from build123d import *

# Parameters (mm, degrees)
BOSS_EXTRUDE1_DEPTH = 13.33
FILLET1_R           = 20
SKETCH3_R           = 3.33
CUT_EXTRUDE2_DEPTH  = 68.320131462
FILLET2_R           = 3.333
SKETCH4_R           = 2.8333333
DOME1_FACE_RADIUS   = 2.8333333
DOME1_HEIGHT        = 3.3333333
CUT_EXTRUDE3_DEPTH  = 2
CUT_EXTRUDE5_DEPTH  = 13.34
SKETCH19_R          = 1.425
CUT_EXTRUDE6_DEPTH  = 8.6


with BuildPart() as part:
    # Sketch1 → Boss-Extrude1 (new body)
    with BuildSketch(Plane(origin=(0, 0, 0), x_dir=(1, 0, 0), z_dir=(0, 1, 0))):
        with BuildLine():
            Line((25.438564969, 21.535280641), (27.993333135, 37.33))
            ThreePointArc((27.993333135, 37.33), (42.371570445, -19.53984693), (-10.216878485, -45.527694802))
            Line((-10.216878485, -45.527694802), (1.110949751, -33.311479863))
            ThreePointArc((1.110949751, -33.311479863), (30.46737546, -13.513990254), (25.438564969, 21.535280641))
        make_face()
    extrude(amount=BOSS_EXTRUDE1_DEPTH)

    # Fillet1
    fillet1_edges = [part.edges().sort_by_distance(p)[0] for p in [
        (1.110949751, 6.665, 33.311479863),
    ]]
    fillet(fillet1_edges, radius=FILLET1_R)

    # Sketch3 → Cut-Extrude2 (cut, through all)
    with BuildSketch(Plane(origin=(0, 13.33, 0), x_dir=(1, 0, 0), z_dir=(0, 1, 0))):
        with Locations(Location((35.289122258, 19.812921474, 0), (0, 0, 270))):
            Circle(SKETCH3_R)
    extrude(amount=-CUT_EXTRUDE2_DEPTH, mode=Mode.SUBTRACT)

    # Fillet2
    fillet2_edges = [part.edges().sort_by_distance(p)[0] for p in [
        (27.993333135, 6.665, -37.33),
    ]]
    fillet(fillet2_edges, radius=FILLET2_R)

    # Sweep1: sweep along a path in Sketch6
    with BuildLine(Plane.XY) as sweep1_path:
        Line((40.567020893, 13.33), (40.567020893, 20.636666))
        ThreePointArc((40.567020893, 20.636666), (45.278451651, 24.683063573), (48.567020893, 19.414645837))
    # Sketch4 → Sweep1 (sweep)
    with BuildSketch(Plane(origin=(0, 13.33, 0), x_dir=(1, 0, 0), z_dir=(0, 1, 0))):
        with Locations((40.567020893, 0.715488074)):
            Circle(SKETCH4_R)
    sweep(path=sweep1_path.line)

    # Dome1: a dome of height H over a round flat face of radius A is a cap of a sphere of radius (A * A + H * H) / (2 * H)
    dome1_r = (DOME1_FACE_RADIUS * DOME1_FACE_RADIUS + DOME1_HEIGHT * DOME1_HEIGHT) / (2 * DOME1_HEIGHT)
    dome1_base = Plane((48.567020893, 19.414645837, -0.715488074), z_dir=(-0.298539128134, -0.954397395728, 0))
    with Locations(dome1_base.offset(DOME1_HEIGHT - dome1_r)):
        dome1_ball = Sphere(dome1_r, mode=Mode.PRIVATE)
    add(split(dome1_ball, bisect_by=dome1_base, keep=Keep.TOP, mode=Mode.PRIVATE))

    # Sketch7 → Cut-Extrude3 (cut, symmetric)
    with BuildSketch(Plane(origin=(0, 6.665, 0), x_dir=(1, 0, 0), z_dir=(0, 1, 0))):
        with BuildLine():
            ThreePointArc((44.965852541, -12.459041105), (45.327303444, -11.072089345), (45.645985213, -9.674690379))
            ThreePointArc((45.645985213, -9.674690379), (41.52914689, -0.997602982), (46.057874066, 7.47180276))
            ThreePointArc((46.057874066, 7.47180276), (45.806657105, 8.882891694), (45.51221871, 10.285599066))
            ThreePointArc((45.51221871, 10.285599066), (38.862616133, -0.933548234), (44.965852541, -12.459041105))
        make_face()
    extrude(amount=CUT_EXTRUDE3_DEPTH, both=True, mode=Mode.SUBTRACT)

    # Sketch18 → Cut-Extrude5 (cut)
    with BuildSketch(Plane.XZ):
        with BuildLine():
            Line((28.039143401, -31.35294351), (26.341104847, -22.015791956))
            ThreePointArc((26.341104847, -22.015791956), (28.034108775, -19.815086303), (29.543730196, -17.484762112))
            ThreePointArc((29.543730196, -17.484762112), (32.195597251, -23.521489799), (38.760601016, -24.1340301))
            ThreePointArc((38.760601016, -24.1340301), (35.637384762, -28.544919116), (32.014856699, -32.555868143))
            ThreePointArc((32.014856699, -32.555868143), (29.659442281, -33.169198731), (28.039143401, -31.35294351))
        make_face()
        with BuildLine():
            Line((18.550254331, 41.721980589), (10.749078367, 32.603776074))
            ThreePointArc((10.749078367, 32.603776074), (16.777611199, 29.950970977), (22.188585816, 26.195716434))
            ThreePointArc((22.188585816, 26.195716434), (27.124492616, 29.226219474), (31.260994101, 33.280412374))
            ThreePointArc((31.260994101, 33.280412374), (25.260742984, 38.035910189), (18.550254331, 41.721980589))
        make_face()
        with BuildLine():
            ThreePointArc((40.820629514, -20.457561098), (36.928571374, -15.146521153), (30.394540812, -15.959974588))
            ThreePointArc((30.394540812, -15.959974588), (33.016991898, -9.403570916), (34.242514373, -2.449307946))
            ThreePointArc((34.242514373, -2.449307946), (39.834796056, -4.973265496), (45.573843855, -2.803632696))
            ThreePointArc((45.573843855, -2.803632696), (44.089869065, -11.870932812), (40.820629514, -20.457561098))
        make_face()
        with BuildLine():
            ThreePointArc((45.651589838, 0.876324867), (39.98520163, 3.873028579), (34.318813422, 0.876324867))
            ThreePointArc((34.318813422, 0.876324867), (33.458600037, 7.685764997), (31.260994101, 14.187993085))
            ThreePointArc((31.260994101, 14.187993085), (36.627069292, 16.498940097), (42.462553984, 16.785919968))
            ThreePointArc((42.462553984, 16.785919968), (44.769458221, 8.973918351), (45.651589838, 0.876324867))
        make_face()
        with BuildLine():
            ThreePointArc((39.931059829, 22.143758962), (35.264351947, 18.298272838), (29.224062449, 18.013968857))
            ThreePointArc((29.224062449, 18.013968857), (26.794540492, 21.461628545), (23.960583625, 24.58534792))
            ThreePointArc((23.960583625, 24.58534792), (27.897400776, 28.917406773), (33.24466644, 31.299005627))
            ThreePointArc((33.24466644, 31.299005627), (36.873111669, 26.929709168), (39.931059829, 22.143758962))
        make_face()
    extrude(amount=-CUT_EXTRUDE5_DEPTH, mode=Mode.SUBTRACT)

    # Sketch19 → Cut-Extrude6 (cut, symmetric)
    with BuildSketch(Plane(origin=(15.613362891, 0, 27.64706404), x_dir=(0.8707413871359999, 0, -0.491741229437267), z_dir=(0.491741229437267, 0, 0.8707413871359999))):
        with Locations(Location((-14.136648815, 6.665, 0), (0, 0, 180))):
            Circle(SKETCH19_R)
    extrude(amount=CUT_EXTRUDE6_DEPTH, both=True, mode=Mode.SUBTRACT)


solid = part.part
CAD build for the part. Positions are in the model's coordinates, mm. A direction names the side the tool comes from. Round coordinates to 2 decimals unless told otherwise and drop trailing zeros. Write each loop counter-clockwise with the first axis right and the second up, starting at its lowest first coordinate (ties: lowest second). Pieces come first, ordered by that corner, then holes. Notation, with made-up numbers: M -15,-16 L 38,-16 A9 cw 38,0 Z; hole C 46.25,54.25 d8. An arc over 180 degrees is marked long. Use a Markdown table: item, result. Add a question column.
1. Pull direction Y, two halves, no side cores. Call faces 4 (the face through (36.55, 6.57, 16.48)), 5 (the face through (5.49, 8.056, 37.841)): released by +Y, released by -Y, zero draft, split by the parting line, or undercut.
2. 3-axis set-ups, long thin cutter, end or side, ignore diameter. For faces 1 (the face through (27.202, 6.572, -26.75)), 2 (the face through (26.23, 6.57, -26.43)), 3 (the face through (41.663, 6.693, -0.447)): which of +Z, -Z, +X, -X, +Y, -Y reach the whole face in a straight line?
3. Slice it at D-D on z = 35.5. Give the number of separate pieces and of enclosed holes in the cut face, then the cut area to 3 significant figures.
4. Slice it at C-C on x = 36.5. Give the cut face in (y, z).
5. Drill centre lines: probe 1 along Z at (x, y) = (36.5, 10); probe 2 along Y at (x, z) = (37, -23.5); probe 3 along Z at (x, y) = (19.5, 3.5). Where is each one in solid material? Low to high.
6. Flat gauge pins, fed straight in: P1, Ø0.5, axis at x = 45, z = 10, coming from the +Y side; P2, Ø8, axis at x = 27, y = 5, coming from the +Z side; P3, Ø10, axis at x = 17.5, y = 5, coming from the -Z side; P4, Ø2, axis at x = 35.5, y = 18, coming from the +Z side. Where does each tip first touch, or does it go through?
7. Slice it at A-A on x = 13. Give the cut face in (y, z).
8. Slice it at B-B on y = 1.5. Give the cut face in (x, z).
Reply:
| question | item | result |
|---|---|---|
| 1 | face 4 | zero draft |
| 1 | face 5 | undercut |
| 2 | face 1 | +Y, -Y |
| 2 | face 2 | -Z, -X, +Y, -Y |
| 2 | face 3 | none |
| 3 | separate pieces | 2 |
| 3 | enclosed holes | 1 |
| 3 | area | 192 mm^2 |
| 4 | outline | M 0,-29.07 L 13.33,-29.07 L 13.33,-27.43 L 0,-27.43 Z; M 0,-24.73 L 13.33,-24.73 L 13.33,-22.91 L 0,-22.91 Z; M 0,-16.71 L 13.33,-16.71 L 13.33,-14.98 L 0,-14.98 Z; M 0,-4.13 L 13.33,-4.13 L 13.33,2.92 L 0,2.92 Z; M 0,16.47 L 13.33,16.47 L 13.33,18.88 L 0,18.88 Z; M 0,27.43 L 13.33,27.43 L 13.33,29.07 L 0,29.07 Z |
| 5 | probe 1 | z = -29.07 to -27.43, -24.73 to -22.91, -16.71 to -14.98, -4.13 to 2.92, 16.47 to 18.88, 27.43 to 29.07 |
| 5 | probe 2 | y = 0 to 13.33 |
| 5 | probe 3 | z = 27.03 to 28.25, 41.29 to 42.39 |
| 6 | P1 | stops at y = 13.33 |
| 6 | P2 | stops at z = 40.6 |
| 6 | P3 | stops at z = 24.59 |
| 6 | P4 | passes through |
| 7 | outline | M 0,30.69 L 13.33,30.69 L 13.33,31.77 L 0,31.77 Z; M 0,35.23 L 13.33,35.23 L 13.33,44.81 L 0,44.81 Z |
| 8 | outline | M -10.22,45.53 L -3.81,38.61 A20 ccw 6.79,32.63 A33.33 cw 25.44,-21.54 L 27.05,-31.47 A3.33 ccw 32.67,-33.32 A46.66 ccw Z; hole M 10.75,32.6 A34.33 cw 22.19,26.2 A25.83 ccw 31.26,33.28 A45.66 ccw 18.55,41.72 Z; hole M 23.96,24.59 A34.33 cw 29.22,18.01 A9.58 ccw 39.93,22.14 A45.66 ccw 33.24,31.3 A14.24 ccw Z; hole M 26.34,-22.02 L 28.04,-31.35 A2.33 ccw 32.01,-32.56 A45.66 ccw 38.76,-24.13 A6.5 cw 29.54,-17.48 A34.33 cw Z; hole M 30.39,-15.96 A6.5 cw 40.82,-20.46 A45.66 ccw 45.57,-2.8 A8.02 cw 34.24,-2.45 A34.33 cw Z; hole M 31.26,14.19 A34.33 cw 34.32,0.88 A6.86 cw 45.65,0.88 A45.66 ccw 42.46,16.79 A16.43 ccw Z; hole C 35.29,-19.81 d6.66 |
